The listing builds one solid part. Answer for the finished solid, in the listing's coordinates (mm). A direction names the side the tool comes from. Give positions to 0.01 mm unless a question says otherwise; leave off trailing zeros. Loops run counter-clockwise (first coordinate to the right, second up) from the corner with the lowest first, then second, coordinate; pieces in that order, holes last. Notation, with made-up numbers: (20, -10.5) - (35, -10.5) arc R28 ccw to (35, 26.5) - close; hole circle Ø3 at (58.5, 16.25). An arc over 180 degrees is marked (long way). One line per item, written item: value. Start each with the question number.
from build123d import *

# Parameters (mm, degrees)
SKETCH_1_W          = 20
SKETCH_1_H          = 5
SKETCH_1_W_2        = 130
SKETCH_1_H_2        = 135
EXTRUDE_1_DEPTH     = 10
SKETCH_2_W          = 160
SKETCH_2_H          = 15
EXTRUDE_2_DEPTH     = 90
SKETCH_3_R          = 38.25
CUT_EXTRUDE_1_DEPTH = 2
FILLET_1_R          = 15
FILLET_2_R          = 15
FILLET_3_R          = 65


with BuildPart() as part:
    # 草图1 → 凸台-拉伸1 (new body)
    with BuildSketch(Plane.XY):
        Polygon((0, 0), (30, 0), (30, -15), (95, -15), (95, -180), (-65, -180), (-65, -15), (0, -15), align=None)
        with Locations((15, -7.5)):
            Rectangle(SKETCH_1_W, SKETCH_1_H, mode=Mode.SUBTRACT)
        with Locations((15, -97.5)):
            Rectangle(SKETCH_1_W_2, SKETCH_1_H_2, mode=Mode.SUBTRACT)
    extrude(amount=EXTRUDE_1_DEPTH)

    # 草图2 → 凸台-拉伸2 (add)
    with BuildSketch(Plane.XY.offset(10)):
        with Locations((15, -172.5)):
            Rectangle(SKETCH_2_W, SKETCH_2_H)
    extrude(amount=EXTRUDE_2_DEPTH)

    # 草图3 → 切除-拉伸1 (cut)
    with BuildSketch(Plane(origin=(0, -165, 0), x_dir=(1, 0, 0), z_dir=(0, 1, 0))):
        with Locations((15, -55)):
            Circle(SKETCH_3_R)
    extrude(amount=-CUT_EXTRUDE_1_DEPTH, mode=Mode.SUBTRACT)

    # 圆角1
    fillet_1_edges = [part.edges().sort_by_distance(p)[0] for p in [
        (-57.5, -165, 10),
        (87.5, -165, 10),
    ]]
    fillet(fillet_1_edges, radius=FILLET_1_R)

    # 圆角2
    fillet_2_edges = [part.edges().sort_by_distance(p)[0] for p in [
        (-50, -165, 17.5),
        (80, -165, 17.5),
    ]]
    fillet(fillet_2_edges, radius=FILLET_2_R)

    # 圆角3
    fillet_3_edges = [part.edges().sort_by_distance(p)[0] for p in [
        (-65, -172.5, 100),
        (95, -172.5, 100),
    ]]
    fillet(fillet_3_edges, radius=FILLET_3_R)


solid = part.part
1. For faces 1 (the flat face through (-33, -15, 5)), 2 (the flat face through (14, -30, 5)), 3 (the flat face through (14, -167, 54)), determine the directions among +Z, -Z, +X, -X, +Y, -Y from which every point of the face is accessible in a straight line to the end or side of a thin tool.
2. A cutting plane is placed at B-B (x = 15). Determine the outline of the cut face in (y, z), plus the area to 3 significant figures.
3. Find the intervals of material crossed by L1, parallel to Z at x = 15, y = -166; L2, parallel to Y at x = 2, z = 37; L3, parallel to Y at x = -30.5, z = 41.5, in increasing order. Write a range as [from, to].
4. A cutting plane is placed at C-C (x = 62.5). Determine the outline of the cut face in (y, z), plus the area to 3 significant figures.
5. A cutting plane is placed at D-D (z = 30.5). Determine the outline of the cut face in (x, y), plus the area to 3 significant figures.
6. A cutting plane is placed at A-A (y = -59.5). Determine the outline of the cut face in (x, z), plus the area to 3 significant figures.
7. Flat-ended cylindrical pins translate along their axes: pin 1 (4 mm diameter, centred on y = -8.5, z = 4.5, fed in from +X); pin 2 (2.5 mm diameter, centred on y = -7.5, z = 3, fed in from -X); pin 3 (8 mm diameter, centred on y = -38, z = 12.5, fed in from +X); pin 4 (8 mm diameter, centred on x = 57, z = 4.5, fed in from +Y). Find the tip coordinate at first contact, or state that the pin passes through.
8. Determine the mould class of faces 4 (the cylindrical face through (6.71, -165.99, 92.34)), 5 (the flat face through (15, 0, 5)), 6 (the cylindrical face through (75.454, -172.395, 81.465)) for opening direction Z: released by +Z, released by -Z, zero draft, split by the parting line, or undercut.
Results below:
1. face 1: +Z, -Z, -X, +Y
1. face 2: +Z, -Z
1. face 3: +Y
2. outline: (-180, 0) - (-165, 0) - (-165, 16.75) - (-167, 16.75) - (-167, 93.25) - (-165, 93.25) - (-165, 100) - (-180, 100) - close; (-30, 0) - (-10, 0) - (-10, 10) - (-30, 10) - close; (-5, 0) - (0, 0) - (0, 10) - (-5, 10) - close
2. area: 1,600 mm^2
3. L1: z = [0, 16.75], [93.25, 100]
3. L2: y = [-180, -167]
3. L3: y = [-180, -165]
4. outline: (-180, 0) - (-165, 0) - (-165, 91.29) - (-180, 91.29) - close; (-30, 0) - (-15, 0) - (-15, 10) - (-30, 10) - close
4. area: 1,520 mm^2
5. outline: (-65, -180) - (95, -180) - (95, -165) - (44.37, -165) - (44.37, -167) - (-14.37, -167) - (-14.37, -165) - (-65, -165) - close
5. area: 2,280 mm^2
6. outline: (-65, 0) - (-50, 0) - (-50, 10) - (-65, 10) - close; (80, 0) - (95, 0) - (95, 10) - (80, 10) - close
6. area: 300 mm^2
7. pin 1: stops at x = 30
7. pin 2: stops at x = 0
7. pin 3: stops at x = 95
7. pin 4: stops at y = -15
8. face 4: undercut
8. face 5: zero draft
8. face 6: released by +Z
